Job drawing, mm, ordinate dimensions from the low corner. One solid piece. A direction names the side the tool comes from. Round coordinates to 2 decimals unless told otherwise and drop trailing zeros. Write each loop counter-clockwise with the first axis right and the second up, starting at its lowest first coordinate (ties: lowest second). Pieces come first, ordered by that corner, then holes. Notation, with made-up numbers: (34, 11.5) - (79, 11.5) arc R23 cw to (79, 37.5) - close; hole circle Ø3 at (-24, -26). An arc over 180 degrees is marked (long way). Write each question's results on one line, items separated by ' | '.
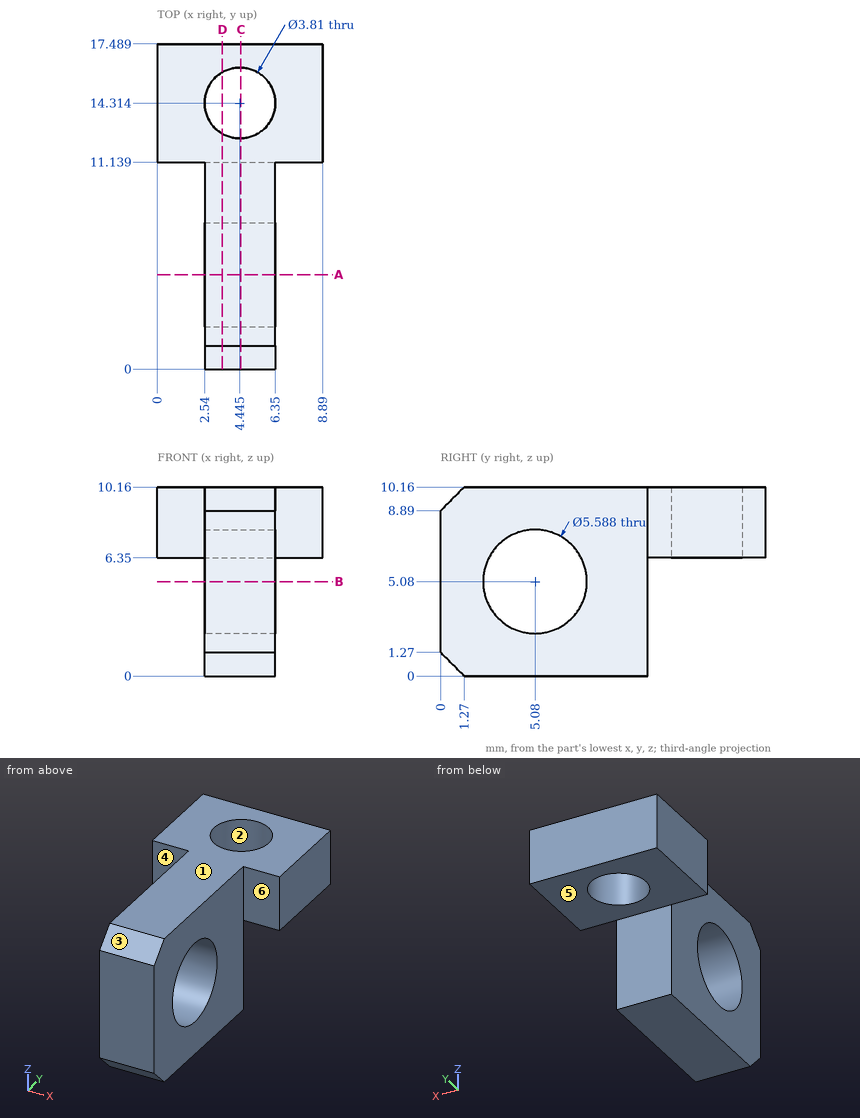
(1) Drill centre lines: probe 1 along Y at (x, z) = (3.95, 5.08); probe 2 along Z at (x, y) = (8, 11.5); probe 3 along X at (y, z) = (10.25, 6.25). Where is each one in solid material? Low to high. Write a range as [from, to].
Worked answers:
probe 1: y = [0, 2.29], [7.87, 11.14] | probe 2: z = [6.35, 10.16] | probe 3: x = [2.54, 6.35]
(2) Flat gauge pins, fed straight in: pin 1 Ø4.5 at (y, z) = (5.08, 5.08) entering from +X; pin 2 Ø1.5 at (x, z) = (3, 1.5) entering from +Y; pin 3 Ø5 at (y, z) = (4, 4.5) entering from -X; pin 4 Ø0.8 at (x, z) = (8, 8) entering from -Y. Where does each tip first touch, or does it go through?
Worked answers:
pin 1: passes through | pin 2: stops at y = 11.14 | pin 3: stops at x = 2.54 | pin 4: stops at y = 11.14
(3) Slice it at C-C, the plane x = 4.5. Write the cut outline in (y, z).
Worked answers:
outline: (0, 1.27) - (1.27, 0) - (11.14, 0) - (11.14, 6.35) - (12.41, 6.35) - (12.41, 10.16) - (1.27, 10.16) - (0, 8.89) - close; (16.22, 6.35) - (17.49, 6.35) - (17.49, 10.16) - (16.22, 10.16) - close; hole circle Ø5.59 at (5.08, 5.08)
(4) Slice it at A-A, the plane y = 5.08. Write the cut outline in (x, z).
Worked answers:
outline: (2.54, 0) - (6.35, 0) - (6.35, 2.29) - (2.54, 2.29) - close; (2.54, 7.87) - (6.35, 7.87) - (6.35, 10.16) - (2.54, 10.16) - close
(5) Slice it at D-D, the plane x = 3.5. Write the cut outline in (y, z).
Worked answers:
outline: (0, 1.27) - (1.27, 0) - (11.14, 0) - (11.14, 6.35) - (12.66, 6.35) - (12.66, 10.16) - (1.27, 10.16) - (0, 8.89) - close; (15.97, 6.35) - (17.49, 6.35) - (17.49, 10.16) - (15.97, 10.16) - close; hole circle Ø5.59 at (5.08, 5.08)
(6) Tool access for the marked faces 4, 5 and 6: list every direction of +Z, -Z, +X, -X, +Y, -Y with a clear straight run to the whole face (end or side of a thin tool).
Worked answers:
face 4: +Z, -Z, -X, -Y | face 5: -Z, +X, -X, +Y | face 6: +Z, -Z, +X, -Y
(7) Two-plate mould, pull along Y, no slides. Class the marked faces 1, 2 and 3: released by +Y, released by -Y, zero draft, split by the parting line, or undercut.
Worked answers:
face 1: zero draft | face 2: undercut | face 3: released by -Y
(8) Slice it at B-B, the plane z = 5.08. Write the cut outline in (x, y).
Worked answers:
outline: (2.54, 0) - (6.35, 0) - (6.35, 2.29) - (2.54, 2.29) - close; (2.54, 7.87) - (6.35, 7.87) - (6.35, 11.14) - (2.54, 11.14) - close
